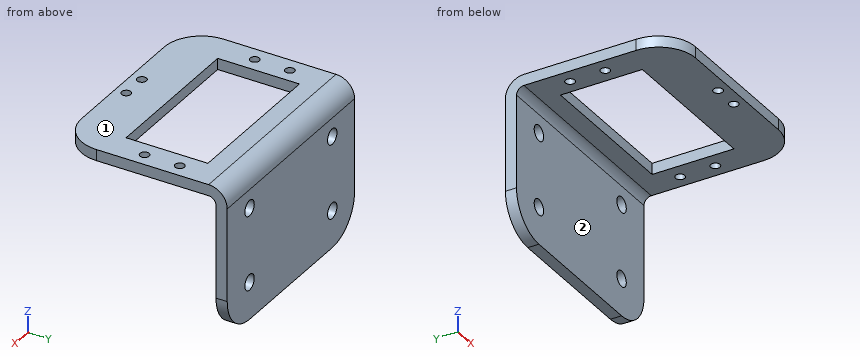
```python
from build123d import *

# Parameters (mm, degrees)
SKETCH_1_W                       = 57
SKETCH_1_H                       = 45.164593648
SKETCH_1_R                       = 1.25
EXTRUDE_1_DEPTH                  = 3
SM_EDGE_FLANGE_1_STRIP_W         = 16
SM_EDGE_FLANGE_1_STRIP_H         = 3
SM_EDGE_FLANGE_1_STRIP_CUT_DEPTH = 57
SM_EDGE_FLANGE_1_DEPTH           = 57
SKETCH_9_R                       = 2.1
CUT_EXTRUDE_1_DEPTH              = 10
FILLET_1_R                       = 10


# Sheet-metal steps are written as plain solids
with BuildPart() as part:
    # Sketch 1 → 填料-伸長1 (new body)
    with BuildSketch(Plane.XY):
        with Locations((28.5, -12.582296824)):
            Rectangle(SKETCH_1_W, SKETCH_1_H)
        Polygon((8, -22), (8, 0), (49, 0), (49, -14.454593648), (49, -22), align=None, mode=Mode.SUBTRACT)
        with Locations((25, -32.164593648)):
            Circle(SKETCH_1_R, mode=Mode.SUBTRACT)
        with Locations((4, -14.454593648)):
            Circle(SKETCH_1_R, mode=Mode.SUBTRACT)
        with Locations((32, -32.164593648)):
            Circle(SKETCH_1_R, mode=Mode.SUBTRACT)
        with Locations((53.25, -14.454593648)):
            Circle(SKETCH_1_R, mode=Mode.SUBTRACT)
        with Locations((4, -5)):
            Circle(SKETCH_1_R, mode=Mode.SUBTRACT)
        with Locations((53.25, -5)):
            Circle(SKETCH_1_R, mode=Mode.SUBTRACT)
    extrude(amount=EXTRUDE_1_DEPTH)

    # 邊線-凸緣1 strip (across the edge) → 邊線-凸緣1 strip cut (cut)
    with BuildSketch(Plane(origin=(0, 10, 0), x_dir=(0, -1, 0), z_dir=(1, 0, 0))):
        with Locations((-3, -1.5)):
            Rectangle(SM_EDGE_FLANGE_1_STRIP_W, SM_EDGE_FLANGE_1_STRIP_H)
    extrude(amount=SM_EDGE_FLANGE_1_STRIP_CUT_DEPTH, mode=Mode.SUBTRACT)

    # 邊線-凸緣1 section (across the edge) → 邊線-凸緣1 (add)
    with BuildSketch(Plane(origin=(0, 10, 0), x_dir=(0, -1, 0), z_dir=(1, 0, 0))):
        with BuildLine():
            Line((0, 2), (0, 37))
            Line((0, 37), (3, 37))
            Line((3, 37), (3, 2))
            ThreePointArc((3, 2), (3.585786438, 0.585786438), (5, 0))
            Line((5, 0), (5, -3))
            ThreePointArc((5, -3), (1.464466094, -1.535533906), (0, 2))
        make_face()
    extrude(amount=SM_EDGE_FLANGE_1_DEPTH)

    # 草圖9 → 除料-伸長1 (cut)
    with BuildSketch(Plane(origin=(0, 7, 0), x_dir=(-1, 0, 0), z_dir=(0, -1, 0))):
        with Locations(Location((-10, 27, 0), (0, 0, 90))):
            Circle(SKETCH_9_R)
        with Locations(Location((-47, 27, 0), (0, 0, 90))):
            Circle(SKETCH_9_R)
        with Locations(Location((-10, 7, 0), (0, 0, 90))):
            Circle(SKETCH_9_R)
        with Locations(Location((-47, 7, 0), (0, 0, 90))):
            Circle(SKETCH_9_R)
    extrude(amount=-CUT_EXTRUDE_1_DEPTH, mode=Mode.SUBTRACT)

    # 圓角1
    fillet_1_edges = [part.edges().sort_by_distance(p)[0] for p in [
        (57, -35.164593648, 1.5),
        (0, -35.164593648, 1.5),
        (0, 8.5, -37),
        (57, 8.5, -37),
    ]]
    fillet(fillet_1_edges, radius=FILLET_1_R)


solid = part.part
```
Work out the finished part from the listing and answer in its coordinate system (mm). Face numbers are marked on the shaded views. A direction names the side the tool comes from. Round coordinates to 2 decimals unless told otherwise and drop trailing zeros. Loops run counter-clockwise (first coordinate to the right, second up) from the corner with the lowest first, then second, coordinate; pieces in that order, holes last. Notation, with made-up numbers: M -18,88.5 L 14,88.5 A14 cw 14,107.5 Z; hole C 53.25,82 d8. An arc over 180 degrees is marked long. One line per question, with ' | ' between items.
Q1. Consider line 1 along Y through (x, z) = (45, -31); line 2 along Z through (x, y) = (48, -25). Determine where each line is inside the solid, lowest interval first. Write a range as from..to.
Conclusion:
line 1: y = 7..10 | line 2: z = 0..3
Q2. A tool of negligible diameter and unlimited length cuts with its end or side. For the marked faces 1 and 2, from which of +Z, -Z, +X, -X, +Y, -Y can it reach the whole face along a straight path? Write none if from no direction.
Conclusion:
face 1: +Z, +X, -X, +Y, -Y | face 2: -Z, +X, -X, -Y
Q3. Find section B-B, the plane z = -7. Give the vertices of the cut face in (x, y), then the cut area to 3 significant figures.
Conclusion:
outline: M 0,7 L 7.9,7 L 7.9,10 L 0,10 Z; M 12.1,7 L 44.9,7 L 44.9,10 L 12.1,10 Z; M 49.1,7 L 57,7 L 57,10 L 49.1,10 Z | area: 146 mm2
Q4. Find section A-A, the plane x = 25. Give the vertices of the cut face in (y, z), then the cut area to 3 significant figures.
Conclusion:
outline: M -35.16,0 L -33.41,0 L -33.41,3 L -35.16,3 Z; M -30.91,0 L -22,0 L -22,3 L -30.91,3 Z; M 0,0 L 5,0 A2 cw 7,-2 L 7,-37 L 10,-37 L 10,-2 A5 ccw 5,3 L 0,3 Z | area: 168 mm2
Q5. Find section C-C, the plane y = -19. Give the vertices of the cut face in (x, z).
Conclusion:
outline: M 0,0 L 8,0 L 8,3 L 0,3 Z; M 49,0 L 57,0 L 57,3 L 49,3 Z
Q6. Each of these flat-tipped pins is pushed along its axis until it touches: pin 1 Ø5 at (x, z) = (10, -7) entering from +Y; pin 2 Ø3 at (x, y) = (32, -32.16) entering from -Z; pin 3 Ø2.5 at (x, z) = (31.5, 2) entering from +Y; pin 4 Ø5 at (x, z) = (25, -5) entering from -Y. Where does it stop, or does it pass through?
Conclusion:
pin 1: stops at y = 10 | pin 2: stops at z = 0 | pin 3: stops at y = 9.18 | pin 4: stops at y = 7
Q7. Find section D-D, the plane z = -21. Give the vertices of the cut face in (x, y).
Conclusion:
outline: M 0,7 L 57,7 L 57,10 L 0,10 Z
